Source: CAD feature listing. Evaluate the final solid. Frame: model axes, mm. Give positions to 0.01 mm unless a question says otherwise; leave off trailing zeros. Loops run counter-clockwise (first coordinate to the right, second up) from the corner with the lowest first, then second, coordinate; pieces in that order, holes last. Notation, with made-up numbers: (-13, -25.5) -> (13, -25.5) arc R19 ccw to (13, -6.5) -> close; hole circle Ø8 at (65.25, -5.5). An arc over 180 degrees is marked (long way). Put each result on its own line as item: value.
Autodesk Inventor part; units mm, degrees
ref_plane "YZ Plane" through (0, 0, 0) normal (1, 0, 0) x (0, 1, 0)
ref_plane "XZ Plane" through (0, 0, 0) normal (0, 1, 0) x (-1, 0, 0)
ref_plane "XY Plane" through (0, 0, 0) normal (0, 0, 1) x (1, 0, 0)
sketch "Эскиз1" plane through (0, 0, 0) normal (0, 0, 1) x (1, 0, 0)
  line L0 (-194.75, 26) -> (-144.75, 26)
  line L1 (-144.75, 26) -> (-144.75, 324)
  line L2 (-144.75, 324) -> (-124.75, 344)
  line L3 (-124.75, 344) -> (125.25, 344)
  line L4 (125.25, 344) -> (145.25, 324)
  line L5 (145.25, 324) -> (145.25, 26)
  line L6 (145.25, 26) -> (195.25, 26)
  line L7 (195.25, 26) -> (195.25, 534)
  line L8 (195.25, 534) -> (-194.75, 534)
  line L9 (-194.75, 534) -> (-194.75, 26)
  circle A0 centre (1.25, 464) radius 20.6
  circle A1 centre (179.75, 255) radius 2
  circle A2 centre (-179.25, 79.5) radius 2
  circle A3 centre (179.75, 40) radius 1.5
  circle A4 centre (-179.25, 337) radius 1.5
  circle A5 centre (-179.25, 40) radius 1.5
  circle A6 centre (-179.25, 308) radius 2
  circle A7 centre (179.75, 292) radius 2
  circle A8 centre (-158.5, 122) radius 1.5
  circle A9 centre (-158.5, 254) radius 1.5
  circle A10 centre (-158.5, 284) radius 1.5
  circle A11 centre (-158.5, 92) radius 1.5
  circle A12 centre (150.5171, 178.4783) radius 1.5
  line L10 (-144.25, 26) -> (144.75, 26)
  line L11 (-124.5429, 343.5) -> (-144.25, 323.7929)
  line L12 (-144.25, 323.7929) -> (-144.25, 26)
  line L13 (-144.25, 25.5) -> (-195.25, 25.5)
  line L14 (-195.25, 25.5) -> (-195.25, 534.5)
  line L15 (-195.25, 534.5) -> (195.75, 534.5)
  line L16 (195.75, 534.5) -> (195.75, 25.5)
  line L17 (195.75, 25.5) -> (144.75, 25.5)
  line L18 (144.75, 26) -> (144.75, 323.7929)
  line L19 (144.75, 323.7929) -> (125.0429, 343.5)
  line L20 (125.0429, 343.5) -> (-124.5429, 343.5)
  circle A13 centre (-130.5, 284) radius 1.5
  circle A14 centre (-130.5, 254) radius 1.5
  circle A15 centre (-130.5, 122) radius 1.5
  circle A16 centre (-130.5, 92) radius 1.5
  dimension "d21" = 0.5
  dimension "d22" = 0.5
  dimension "d23" = 0.5
  dimension "d24" = 0.5
extrude "Выдавливание1" add sketch "Эскиз1" against normal blind 4 contours L12 L11 L20 L19 L18 L10
sketch "Эскиз2" plane through (0, 0, 0) normal (0, 0, 1) x (1, 0, 0)
  circle A0 centre (-130.5, 92) radius 1.5
  circle A1 centre (-130.5, 122) radius 1.5
  circle A2 centre (-130.5, 254) radius 1.5
  circle A3 centre (-130.5, 284) radius 1.5
  line L0 (-114.5429, 343.5) -> (-144.25, 313.7929)
  line L1 (-144.25, 313.7929) -> (-144.25, 43.1688)
  line L2 (-144.25, 43.1688) -> (-103.3546, -10.5)
  line L3 (-103.3546, -10.5) -> (103.8544, -10.5)
  line L4 (103.8544, -10.5) -> (144.75, 43.1637)
  line L5 (144.75, 43.1637) -> (144.75, 313.7929)
  line L6 (144.75, 313.7929) -> (115.0429, 343.5)
  line L7 (115.0429, 343.5) -> (-114.5429, 343.5)
  line L8 (144.75, 43.1637) -> (144.75, 313.7929)
  line L9 (144.75, 178.4783) -> (129.75, 178.4783)
  line L10 (129.75, 178.4783) -> (129.75, 188.4783)
  circle A4 centre (129.75, 188.4783) radius 1.5
  circle A5 centre (129.75, 168.4783) radius 1.5
  point P0 (0, 0)
  dimension "d7" = 3
  dimension "d8" = 3
  dimension "d9" = 10
  dimension "d10" = 20
  dimension "d11" = 15
extrude "Выдавливание2" cut sketch "Эскиз2" against normal blind 10 contours A4 | A5
sketch "Эскиз4" plane through (0, 0, 0) normal (0, 0, 1) x (1, 0, 0)
  line L0 (-106.1226, 31) -> (-137.405, 31)
  line L1 (137.905, 31) -> (106.6226, 31)
  line L2 (-103.3546, -10.5) -> (-144.25, 43.1688)
  line L3 (-134.9774, 31) -> (135.4804, 31)
  line L4 (144.75, 43.1637) -> (103.8544, -10.5)
  line L5 (-103.3546, -10.5) -> (103.8544, -10.5)
  line L6 (-134.9774, 31) -> (-103.3546, -10.5)
  line L7 (-103.3546, -10.5) -> (103.8544, -10.5)
  line L8 (103.8544, -10.5) -> (135.4804, 31)
  line L9 (-131.1675, 26) -> (131.67, 26)
  point P0 (0, 0)
  dimension "d16" = 0
  dimension "d19" = 12.1688
  dimension "d20" = 5
extrude "Выдавливание4" cut sketch "Эскиз4" against normal blind 5 contours L9 L4 L5 L2
sketch "Эскиз7" plane through (0, 0, 0) normal (0, 0, 1) x (1, 0, 0)
  line L0 (-131.9699, 31.6699) -> (-66.8244, 65.3301) construction
  line L1 (-64.0309, 66) -> (0.25, 66) construction
  line L2 (0.25, 65.3301) -> (57.2313, 65.3301) construction
  line L3 (59.4686, 65.3301) -> (67.3244, 65.3301) construction
  line L4 (67.3244, 65.3301) -> (132.4699, 31.6699) construction
  line L5 (144.9404, 31) -> (68.8214, 70.3301) construction
  line L6 (-144.4404, 31) -> (-68.3214, 70.3301) construction
  line L7 (0.25, 71) -> (-65.5279, 71) construction
  line L8 (66.0279, 71) -> (0.25, 71) construction
  line L9 (-144.25, 26) -> (144.75, 26)
  line L10 (-134.2295, 26) -> (-64.5556, 62)
  line L11 (-64.5556, 62) -> (65.0556, 62)
  line L12 (65.0556, 62) -> (134.7295, 26)
  line L13 (134.7295, 26) -> (-134.2295, 26)
  line L14 (-144.25, 323.7929) -> (-144.25, 26)
  line L15 (144.75, 323.7929) -> (144.75, 26)
  point P0 (0, 0)
  dimension "d32" = 4
  dimension "d33" = 4
  dimension "d34" = 4
extrude "Выдавливание6" cut sketch "Эскиз7" against normal blind 5
properties part number "дверька"
(1) Draft query along X for faces 1 (the flat face through (-2, 187, 0)), 2 (the flat face through (99.405, 44.252, -1.972)), 3 (the flat face through (135.034, 333.509, -1.972)), 4 (the flat face through (-99.88, 43.75, -1.97)). Return one class per face: released by +X, released by -X, zero draft, split by the parting line, or undercut.
Calculated:
face 1: zero draft
face 2: undercut
face 3: released by +X
face 4: undercut
(2) First-contact query: P1, Ø2.5, axis at x = 129.75, y = 188.48, coming from the -Z side; P2, Ø1.2, axis at x = -15, z = -2.5, coming from the -Y side. Flat tips, straight axial feed; report the tip coordinate or a pass-through.
Calculated:
P1: passes through
P2: stops at y = 62
(3) Section C-C on x = -77.5. Return loops of the section in (y, z).
Calculated:
outline: (55.31, -4) -> (343.5, -4) -> (343.5, 0) -> (55.31, 0) -> close
(4) Line query: probe 1 along X at (y, z) = (92, -3.15); probe 2 along Y at (x, z) = (129.75, -3.2); probe 3 along Y at (x, z) = (-30, -2.85). Output: solid intervals per line, ascending. Write a range as from..to.
Calculated:
probe 1: x = -144.25..-132, -129..144.75
probe 2: y = 28.57..166.98, 169.98..186.98, 189.98..338.79
probe 3: y = 62..343.5
(5) Section B-B on x = -31. Return loops of the section in (y, z), then the cut area to 3 significant figures.
Calculated:
outline: (62, -4) -> (343.5, -4) -> (343.5, 0) -> (62, 0) -> close
area: 1,130 mm²
(6) Section A-A on z = -0.6. Return loops of the section in (x, y).
Calculated:
outline: (-144.25, 26) -> (-134.23, 26) -> (-64.56, 62) -> (65.06, 62) -> (134.73, 26) -> (144.75, 26) -> (144.75, 323.79) -> (125.04, 343.5) -> (-124.54, 343.5) -> (-144.25, 323.79) -> close; hole circle Ø3 at (-130.5, 92); hole circle Ø3 at (-130.5, 122); hole circle Ø3 at (-130.5, 254); hole circle Ø3 at (-130.5, 284); hole circle Ø3 at (129.75, 168.48); hole circle Ø3 at (129.75, 188.48)
